from build123d import *

# Parameters (mm, degrees)
F0_R     = 12.7
F1_DEPTH = 12.7
F2_R     = 5.08
F3_R     = 6.5
F4_DEPTH = 5
F5_R     = 12.7
F6_DEPTH = 12.7
F7_R     = 5.08
F9_D     = 8.5


with BuildPart() as f1:
    # F0 (on Front) → F1 (new body)
    with BuildSketch(Plane.XZ):
        Circle(F0_R)
    extrude(amount=F1_DEPTH)

    # F2
    f2_edges = [f1.edges().sort_by_distance(p)[0] for p in [
        (-12.7, 0, 0),
        (-12.7, -12.7, 0),
    ]]
    fillet(f2_edges, radius=F2_R)

    # F3 (on Front) → F4 (join)
    with BuildSketch(Plane.XZ):
        Circle(F3_R)
    extrude(amount=-F4_DEPTH)

    # F5 (on face) → F6 (join)
    with BuildSketch(Plane(origin=(0, 5, 0), x_dir=(-1, 0, 0), z_dir=(0, 1, 0))):
        Circle(F5_R)
    extrude(amount=F6_DEPTH)

    # F7
    f7_edges = [f1.edges().sort_by_distance(p)[0] for p in [
        (12.7, 17.7, 0),
        (12.7, 5, 0),
    ]]
    fillet(f7_edges, radius=F7_R)

    # F9 (through all)
    with Locations(Plane(origin=(0, 17.7, 0), x_dir=(-1, 0, 0), z_dir=(0, 1, 0))):
        with Locations((0, 0)):
            Hole(F9_D / 2)


solid = f1.part
Here's how the part is built. I have some questions about the finished solid (model axes, mm). A direction names the side the tool comes from. Round coordinates to 2 decimals unless told otherwise and drop trailing zeros. Write each loop counter-clockwise with the first axis right and the second up, starting at its lowest first coordinate (ties: lowest second). Pieces come first, ordered by that corner, then holes.
1. Suppose I cut it at B-B (x = 0). List the corners of the cut face in (y, z) for me.
2. Will these pins go through, and if not, where does the flat tip stop? pin 1 Ø5 at (x, y) = (-9, -1.5) entering from -Z; pin 2 Ø8 at (y, z) = (3, -6.5) entering from +X; pin 3 Ø8 at (y, z) = (0, 1) entering from -X.
3. Suppose I cut it at A-A (z = 0). List the corners of the cut face in (x, y) for me, and give its area (3 significant figures).
4. For faces 1 (the cylindrical face through (-5.158, 2.465, -3.955)), 2 (the cylindrical face through (2.75, 11.33, -12.4)), which set-ups out of +Z, -Z, +X, -X, +Y, -Y let a thin tool reach every point of the face, with its end or its side?
5. If we mould it in two halves opening along Y, with no side actions, what happens to faces 3 (the flat face through (-3.3, 17.7, -3.3)), 4 (the flat face through (6, 0, 3)), 5 (the cylindrical face through (2.285, 2.287, 3.584))? For each: released by +Y, released by -Y, zero draft, split by the parting line, or undercut.
6. I need wall thicknesses on L1, parallel to Z at x = 0, y = 4; L2, parallel to Z at x = 0, y = -6; L3, parallel to Y at x = 0.75, z = 7.25. Which ranges of each line are inside material? Lowest first, please.
7. Suppose I cut it at C-C (y = 1.5). List the corners of the cut face in (x, z) for me.
8. Suppose I cut it at D-D (y = -5.5). List the corners of the cut face in (x, z) for me, and give its area (3 significant figures).
Answer sheet:
1. outline: (-12.7, -7.62) arc R5.08 ccw to (-7.62, -12.7) - (-5.08, -12.7) arc R5.08 ccw to (0, -7.62) - (0, -6.5) - (5, -6.5) - (5, -7.62) arc R5.08 ccw to (10.08, -12.7) - (12.62, -12.7) arc R5.08 ccw to (17.7, -7.62) - (17.7, -4.25) - (-12.7, -4.25) - close; (-12.7, 4.25) - (17.7, 4.25) - (17.7, 7.62) arc R5.08 ccw to (12.62, 12.7) - (10.08, 12.7) arc R5.08 ccw to (5, 7.62) - (5, 6.5) - (0, 6.5) - (0, 7.62) arc R5.08 ccw to (-5.08, 12.7) - (-7.62, 12.7) arc R5.08 ccw to (-12.7, 7.62) - close
2. pin 1: stops at z = -10.06
2. pin 2: stops at x = 10.27
2. pin 3: stops at x = -12.57
3. outline: (-12.7, -7.62) arc R5.08 ccw to (-7.62, -12.7) - (-4.25, -12.7) - (-4.25, 17.7) - (-7.62, 17.7) arc R5.08 ccw to (-12.7, 12.62) - (-12.7, 10.08) arc R5.08 ccw to (-7.62, 5) - (-6.5, 5) - (-6.5, 0) - (-7.62, 0) arc R5.08 ccw to (-12.7, -5.08) - close; (4.25, -12.7) - (7.62, -12.7) arc R5.08 ccw to (12.7, -7.62) - (12.7, -5.08) arc R5.08 ccw to (7.62, 0) - (6.5, 0) - (6.5, 5) - (7.62, 5) arc R5.08 ccw to (12.7, 10.08) - (12.7, 12.62) arc R5.08 ccw to (7.62, 17.7) - (4.25, 17.7) - close
3. area: 407 mm2
4. face 1: none
4. face 2: +Y, -Y
5. face 3: released by +Y
5. face 4: undercut
5. face 5: zero draft
6. L1: z = -6.5 to -4.25, 4.25 to 6.5
6. L2: z = -12.7 to -4.25, 4.25 to 12.7
6. L3: y = -12.7 to 0, 5 to 17.7
7. outline: circle Ø13 at (0, 0); hole circle Ø8.5 at (0, 0)
8. outline: circle Ø25.4 at (0, 0); hole circle Ø8.5 at (0, 0)
8. area: 450 mm2
